Can you work these out from the model? Positions are in its coordinate system, mm. A direction names the side the tool comes from. Coordinates: 2 decimals unless noted, no trailing zeros. Order: outer loops, then holes, each group sorted by start corner. A loop starts at its lowest first (then second) coordinate and runs counter-clockwise, first axis right, second up. Notation, with made-up numbers: (-5, -17) -> (0, -17) arc R4 cw to (0, -12) -> close; hole circle Ø2 at (74.25, 81). An arc over 180 degrees is marked (long way). Use a Markdown table: item, result. Add a question column.
1. For faces 4 (the flat face through (-127, -30, 6)), 5 (the flat face through (-79, -69, 0)), 6 (the flat face through (-84, -120, 4)), which set-ups out of +Z, -Z, +X, -X, +Y, -Y let a thin tool reach every point of the face, with its end or its side?
2. Suppose I cut it at C-C, the plane z = 9. State how many separate pieces and enclosed holes the cut face has, then the cut area to 3 significant figures.
3. We'd pull the mould along Y, two halves only. Please class faces 1 (the flat face through (-132, -20, 4)), 2 (the cylindrical face through (-86.59, -75.34, 5.92)), 3 (the flat face through (-20, -103, 4)): pulls with the +Y half, pulls with the -Y half, needs draft (parallel to the pull), parting line crosses it, or undercut.
4. For pin 1 Ø8 at (x, z) = (-95.5, 5.5) entering from +Y; pin 2 Ø5 at (y, z) = (-63.5, 4) entering from +X, each with a flat end and sliding along its axis, tell me the tip position at first contact or that it passes through.
5. Suppose I cut it at A-A, the plane y = -98. List the corners of the cut face in (x, z) for me, then the cut area to 3 significant figures.
6. If I drill on line 1 along X through (y, z) = (-110, -0.5); line 2 along Y through (x, z) = (-140, 2); line 3 along X through (y, z) = (-108, 2.25), over which ranges is the centre line in solid material (lowest first)? Write a range as from..to.
7. Suppose I cut it at B-B, the plane x = -140. List the corners of the cut face in (y, z) for me.
```python
from build123d import *

# Parameters (mm, degrees)
F1_DEPTH  = 12
F2_W      = 130
F2_H      = 20
F3_DEPTH  = 5
F4_W      = 105
F4_H      = 20
F5_DEPTH  = 5
F7_W      = 20
F7_H      = 100
F7_R      = 2.5
F7_H_2    = 20
F7_W_2    = 130
F8_DEPTH  = 25
F9_DEPTH  = 5
F10_W     = 130
F10_H     = 20
F10_W_2   = 20
F10_H_2   = 100
F11_DEPTH = 25
F12_W     = 100
F12_H     = 9
F13_DEPTH = 150
F15_DEPTH = 25


with BuildPart() as f1:
    # F0 (on Top) → F1 (new body)
    with BuildSketch(Plane.XY):
        with BuildLine():
            add(Edge.make_bspline(
                [(-116.5, 0), (-116.5, -86.5), (0, -86.5)],
                knots=[3.1415926536, 3.1415926536, 3.1415926536, 4.7123889804, 4.7123889804, 4.7123889804], degree=2, weights=[1, 0.7071067812, 1]))
            Line((-116.5, 0), (-116.5, -86.5))
            Line((-116.5, -86.5), (0, -86.5))
        make_face()
        Polygon((-116.5, -86.5), (-116.5, 0), (-130, 0), (-130, -100), (0, -100), (0, -86.5), align=None)
    extrude(amount=F1_DEPTH)

    # F2 (on face) → F3 (join)
    with BuildSketch(Plane.XZ.offset(100)):
        with Locations((-65, 6)):
            Rectangle(F2_W, F2_H)
    extrude(amount=F3_DEPTH)

    # F4 (on face) → F5 (join)
    with BuildSketch(Plane(origin=(-130, 0, 0), x_dir=(0, -1, 0), z_dir=(-1, 0, 0))):
        with Locations((52.5, 6)):
            Rectangle(F4_W, F4_H)
    extrude(amount=F5_DEPTH)

    # F7 (on face) → F8 (join)
    with BuildSketch(Plane(origin=(0, 0, -4), x_dir=(1, 0, 0), z_dir=(0, 0, -1))):
        with Locations((-140, 50)):
            Rectangle(F7_W, F7_H)
        with Locations((-140, 30)):
            Circle(F7_R, mode=Mode.SUBTRACT)
        with Locations((-140, 80)):
            Circle(F7_R, mode=Mode.SUBTRACT)
        with Locations((-140, 110)):
            Rectangle(F7_W, F7_H_2)
        with Locations((-65, 110)):
            Rectangle(F7_W_2, F7_H_2)
        with Locations((-105, 110)):
            Circle(F7_R, mode=Mode.SUBTRACT)
        with Locations((-30, 110)):
            Circle(F7_R, mode=Mode.SUBTRACT)
    extrude(amount=-F8_DEPTH)

    # F6 (on face) → F9 (join)
    with BuildSketch(Plane.XY.offset(16)):
        Polygon((-120, 0), (-135, 0), (-135, -105), (0, -105), (0, -90), (-120, -90), align=None)
    extrude(amount=F9_DEPTH)

    # F10 (on Top) → F11 (cut, symmetric)
    with BuildSketch(Plane.XY):
        with Locations((-85, -10)):
            Rectangle(F10_W, F10_H)
        with Locations((-10, -10)):
            Rectangle(F10_W_2, F10_H)
        with Locations((-10, -70)):
            Rectangle(F10_W_2, F10_H_2)
    extrude(amount=F11_DEPTH, both=True, mode=Mode.SUBTRACT)

    # F12 (on face) → F13 (cut)
    with BuildSketch(Plane.YZ.offset(-20)):
        with Locations((-70, 16.5)):
            Rectangle(F12_W, F12_H)
    extrude(amount=-F13_DEPTH, mode=Mode.SUBTRACT)

    # F14 (on face) → F15 (cut)
    with BuildSketch(Plane(origin=(0, 0, 0), x_dir=(1, 0, 0), z_dir=(0, 0, -1))):
        with BuildLine():
            Line((-30, 100), (-130, 100))
            Line((-130, 100), (-130, 30))
            Line((-130, 30), (-123.3431933691, 30))
            ThreePointArc((-123.3431933691, 30), (-85.9046810739, 75.8231903114), (-30, 95.2158076494))
            Line((-30, 95.2158076494), (-30, 100))
        make_face()
    extrude(amount=-F15_DEPTH, mode=Mode.SUBTRACT)


solid = f1.part
```
Worked out:
| question | item | result |
|---|---|---|
| 1 | face 4 | +Z, -Z |
| 1 | face 5 | -Z, +X, +Y |
| 1 | face 6 | +Z, -Z, +X, -X, -Y |
| 2 | separate pieces | 1 |
| 2 | enclosed holes | 5 |
| 2 | area | 5,920 mm² |
| 3 | face 1 | pulls with the +Y half |
| 3 | face 2 | undercut |
| 3 | face 3 | needs draft |
| 4 | pin 1 | stops at y = -44.99 |
| 4 | pin 2 | stops at x = -75.3 |
| 5 | outline | (-150, -4) -> (-130, -4) -> (-130, 12) -> (-150, 12) -> close; (-30, 0) -> (-20, 0) -> (-20, 12) -> (-30, 12) -> close |
| 5 | area | 440 mm² |
| 6 | line 1 | x = -150..-107.5, -102.5..-32.5, -27.5..-20 |
| 6 | line 2 | y = -120..-82.5, -77.5..-32.5, -27.5..-20 |
| 6 | line 3 | x = -150..-106.5, -103.5..-31.5, -28.5..-20 |
| 7 | outline | (-120, -4) -> (-82.5, -4) -> (-82.5, 12) -> (-120, 12) -> close; (-77.5, -4) -> (-32.5, -4) -> (-32.5, 12) -> (-77.5, 12) -> close; (-27.5, -4) -> (-20, -4) -> (-20, 12) -> (-27.5, 12) -> close |
